Build history of the part. All positions in model axes, mm. A direction names the side the tool comes from. Give positions to 0.01 mm unless a question says otherwise; leave off trailing zeros. Write each loop counter-clockwise with the first axis right and the second up, starting at its lowest first coordinate (ties: lowest second). Pieces come first, ordered by that corner, then holes. Notation, with made-up numbers: (-23.75, 64.5) -> (22.25, 64.5) arc R21 ccw to (22.25, 85.5) -> close; hole circle Ø7 at (70.25, 25.5). An arc over 180 degrees is marked (long way). Write item = value, one per line. Start each with the question number.
Q1. Wall check: line 1 (Z direction, x = -7, y = -3); line 2 (Y direction, x = -0.25, z = 3.7); line 3 (X direction, y = 2.5, z = 5.7). Give the ranges that are in metal, low to high.
Q2. Tool access for faces 1 (the face through (0, 0, 0)), 2 (the face through (-2, 4, 3)): list every direction of +Z, -Z, +X, -X, +Y, -Y with a clear straight run to the whole face (end or side of a thin tool).
Q3. Saw through at C-C, the plane z = 4.9. List the corners of the cut face in (x, y), then the cut area to 3 significant figures.
Q4. Mould opens along Y. For faces 3 (the face through (4, -4, 2)), 4 (the face through (-0.9, -4.05, 4.48)) say: pulls with the +Y half, pulls with the -Y half, needs draft (parallel to the pull), parting line crosses it, or undercut.
Q5. Drop flat-ended pins along their axis: P1, Ø8, axis at x = 5, y = -8, coming from the -Z side; P2, Ø3, axis at x = -8, y = 0, coming from the +Z side. Give the stop position or say it passes through.
from build123d import *

# Parameters (mm, degrees)
F0_R     = 10.5
F1_DEPTH = 2
F2_R     = 5
F3_DEPTH = 1
F4_R     = 4.15
F5_DEPTH = 3
F6_SIZE2 = 0.5
F6_SIZE  = 2
F7_R     = 1.49999


# Not quite as in the source:
# - a fillet or chamfer is up to 0.001 mm smaller than in the source, because OpenCascade refuses the exact size


with BuildPart() as f1:
    # F0 (on Top) → F1 (new body)
    with BuildSketch(Plane.XY):
        Circle(F0_R)
    extrude(amount=F1_DEPTH)

    # F2 (on face) → F3 (join)
    with BuildSketch(Plane.XY.offset(2)):
        Circle(F2_R)
    extrude(amount=F3_DEPTH)

    # F4 (on face) → F5 (join)
    with BuildSketch(Plane.XY.offset(3)):
        Circle(F4_R)
    extrude(amount=F5_DEPTH)

    # F6
    f6_edges = [f1.edges().sort_by_distance(p)[0] for p in [
        (-10.5, 0, 2),
    ]]
    f6_side = f1.faces().sort_by_distance((-10.203015, 0, 2))[0]
    chamfer(f6_edges, length=F6_SIZE, length2=F6_SIZE2, reference=f6_side)

    # F7 (radius 1.5 in the source; OpenCascade refuses exactly that, so slightly less here)
    f7_edges = [f1.edges().sort_by_distance(p)[0] for p in [
        (-10.5, 0, 0),
    ]]
    fillet(f7_edges, radius=F7_R)


solid = f1.part
Report:
q1.line_1 = 0 to 2
q1.line_2 = -4.14 to 4.14
q1.line_3 = -3.31 to 3.31
q2.face_1 = -Z, +X, -X, +Y, -Y
q2.face_2 = +Z
q3.outline = circle Ø8.3 at (0, 0)
q3.area = 54.1 mm2
q4.face_3 = needs draft
q4.face_4 = parting line crosses it
q5.P1 = 0
q5.P2 = 2
